from build123d import *
from build123d.topology import SkipClean

# Parameters (mm, degrees)
SKETCH1_W               = 112
SKETCH1_H               = 35.5
BOSS_EXTRUDE1_DEPTH     = 1
SKETCH2_W               = 6
SKETCH2_H               = 6
BOSS_EXTRUDE2_DEPTH     = 2
SKETCH3_R               = 1.1
CUT_EXTRUDE1_DEPTH      = 59.822295943
SKETCH4_R               = 2
CUT_EXTRUDE2_DEPTH      = 2
SKETCH5_W               = 20
SKETCH5_H               = 14
CUT_EXTRUDE3_DEPTH      = 59.822295943
CHAMFER1_SIZE           = 0.4
CUT_EXTRUDE4_DEPTH      = 0.2
SKETCH7_W               = 2.2
SKETCH7_H               = 2.2
CUT_EXTRUDE5_DEPTH      = 0.2
MIRROR2_COPY_1_DEPTH    = 0.2
MIRROR2_COPY_2_SKETCH_W = 2.2
MIRROR2_COPY_2_SKETCH_H = 2.2
MIRROR2_COPY_2_DEPTH    = 0.2
CUT_EXTRUDE6_DEPTH      = 59.779779687
CUT_EXTRUDE6_DEPTH_BACK = 59.779779687
SKETCH8_W               = 0.4
SKETCH8_H               = 35.5


with BuildPart() as part:
    # Sketch1 → Boss-Extrude1 (new body)
    with BuildSketch(Plane.XY):
        Rectangle(SKETCH1_W, SKETCH1_H)
    extrude(amount=BOSS_EXTRUDE1_DEPTH)

    # Sketch2 → Boss-Extrude2 (add)
    with BuildSketch(Plane.XY.offset(1)):
        with Locations((-53, 14.75)):
            Rectangle(SKETCH2_W, SKETCH2_H)
        with Locations((-53, -14.75)):
            Rectangle(SKETCH2_W, SKETCH2_H)
        with Locations((53, -14.75)):
            Rectangle(SKETCH2_W, SKETCH2_H)
        with Locations((53, 14.75)):
            Rectangle(SKETCH2_W, SKETCH2_H)
    extrude(amount=BOSS_EXTRUDE2_DEPTH)

    # Sketch3 → Cut-Extrude1 (cut, through all)
    with BuildSketch(Plane.XY.offset(3)):
        with Locations((-53, 14.75)):
            Circle(SKETCH3_R)
        with Locations(Location((-53, -14.75, 0), (0, 0, 180))):
            Circle(SKETCH3_R)
        with Locations((53, -14.75)):
            Circle(SKETCH3_R)
        with Locations(Location((53, 14.75, 0), (0, 0, 180))):
            Circle(SKETCH3_R)
    extrude(amount=-CUT_EXTRUDE1_DEPTH, mode=Mode.SUBTRACT)

    # Sketch4 → Cut-Extrude2 (cut)
    with BuildSketch(Plane(origin=(0, 0, 0), x_dir=(-1, 0, 0), z_dir=(0, 0, -1))):
        with Locations((-53, 14.75)):
            Circle(SKETCH4_R)
        with Locations((-53, -14.75)):
            Circle(SKETCH4_R)
        with Locations((53, 14.75)):
            Circle(SKETCH4_R)
        with Locations((53, -14.75)):
            Circle(SKETCH4_R)
    extrude(amount=-CUT_EXTRUDE2_DEPTH, mode=Mode.SUBTRACT)

    # Sketch5 → Cut-Extrude3 (cut, through all)
    with BuildSketch(Plane(origin=(0, 0, 0), x_dir=(-1, 0, 0), z_dir=(0, 0, -1))):
        with Locations((29.95, 6.75)):
            Rectangle(SKETCH5_W, SKETCH5_H)
    extrude(amount=-CUT_EXTRUDE3_DEPTH, mode=Mode.SUBTRACT)

    # Chamfer1
    chamfer1_edges = [part.edges().sort_by_distance(p)[0] for p in [
        (-39.95, 6.75, 0),
        (-29.95, 13.75, 0),
        (-19.95, 6.75, 0),
        (-29.95, -0.25, 0),
    ]]
    chamfer(chamfer1_edges, length=CHAMFER1_SIZE)

    # Sketch6 → Cut-Extrude4 (cut)
    with SkipClean():  # the faces are left unmerged after this step: merging them gives an invalid solid
        with BuildSketch(Plane(origin=(0, 0, 2), x_dir=(-1, 0, 0), z_dir=(0, 0, -1))):
            with BuildLine():
                Line((-54.1, 13.079670691), (-54.1, 16.420329309))
                ThreePointArc((-54.1, 16.420329309), (-53, 16.75), (-51.9, 16.420329309))
                Line((-51.9, 16.420329309), (-51.9, 13.079670691))
                ThreePointArc((-51.9, 13.079670691), (-53, 12.75), (-54.1, 13.079670691))
            make_face()
        cut_extrude4 = extrude(amount=-CUT_EXTRUDE4_DEPTH, mode=Mode.SUBTRACT)

    # Sketch7 → Cut-Extrude5 (cut)
    with SkipClean():  # the faces are left unmerged after this step: merging them gives an invalid solid
        with BuildSketch(Plane(origin=(0, 0, 2.2), x_dir=(-1, 0, 0), z_dir=(0, 0, -1))):
            with Locations((-53, 14.75)):
                Rectangle(SKETCH7_W, SKETCH7_H)
        cut_extrude5 = extrude(amount=-CUT_EXTRUDE5_DEPTH, mode=Mode.SUBTRACT)

    # Mirror1: Cut-Extrude4, Cut-Extrude5 across plane
    with SkipClean():  # the faces are left unmerged after this step: merging them gives an invalid solid
        add(cut_extrude4.mirror(Plane(origin=(0, 0, 0), x_dir=(0, 0, 1), z_dir=(1, 0, 0))), mode=Mode.SUBTRACT)
        add(cut_extrude5.mirror(Plane(origin=(0, 0, 0), x_dir=(0, 0, 1), z_dir=(1, 0, 0))), mode=Mode.SUBTRACT)

    # Mirror2: Cut-Extrude4, Cut-Extrude5 across plane
    with SkipClean():  # the faces are left unmerged after this step: merging them gives an invalid solid
        add(cut_extrude4.mirror(Plane.ZX), mode=Mode.SUBTRACT)
        add(cut_extrude5.mirror(Plane.ZX), mode=Mode.SUBTRACT)

    # Mirror2 copy 1 sketch → Mirror2 copy 1 (cut)
    with SkipClean():  # the faces are left unmerged after this step: merging them gives an invalid solid
        with BuildSketch(Plane(origin=(0, 0, 2), x_dir=(1, 0, 0), z_dir=(0, 0, -1))):
            with BuildLine():
                Line((-54.1, 13.079670691), (-54.1, 16.420329309))
                ThreePointArc((-54.1, 16.420329309), (-53, 16.75), (-51.9, 16.420329309))
                Line((-51.9, 16.420329309), (-51.9, 13.079670691))
                ThreePointArc((-51.9, 13.079670691), (-53, 12.75), (-54.1, 13.079670691))
            make_face()
        extrude(amount=-MIRROR2_COPY_1_DEPTH, mode=Mode.SUBTRACT)

    # Mirror2 copy 2 sketch → Mirror2 copy 2 (cut)
    with SkipClean():  # the faces are left unmerged after this step: merging them gives an invalid solid
        with BuildSketch(Plane(origin=(0, 0, 2.2), x_dir=(1, 0, 0), z_dir=(0, 0, -1))):
            with Locations((-53, 14.75)):
                Rectangle(MIRROR2_COPY_2_SKETCH_W, MIRROR2_COPY_2_SKETCH_H)
        extrude(amount=-MIRROR2_COPY_2_DEPTH, mode=Mode.SUBTRACT)

    # Sketch8 → Cut-Extrude6 (cut, two sides: drawn at the far end of the back side and taken through both)
    with SkipClean():  # the faces are left unmerged after this step: merging them gives an invalid solid
        with BuildSketch(Plane.XY.offset(1).offset(-CUT_EXTRUDE6_DEPTH_BACK)):
            with Locations((-55.8, 0)):
                Rectangle(SKETCH8_W, SKETCH8_H)
            with Locations((55.8, 0)):
                Rectangle(SKETCH8_W, SKETCH8_H)
        extrude(amount=CUT_EXTRUDE6_DEPTH + CUT_EXTRUDE6_DEPTH_BACK, mode=Mode.SUBTRACT)


solid = part.part
Could you check a few things on this model? Use its own coordinates, in mm. A direction names the side the tool comes from. Coordinates: 2 decimals unless noted, no trailing zeros. Order: outer loops, then holes, each group sorted by start corner. A loop starts at its lowest first (then second) coordinate and runs counter-clockwise, first axis right, second up. Notation, with made-up numbers: (50.25, -28) - (90.25, -28) arc R24 cw to (90.25, 2) - close; hole circle Ø6 at (8.5, 76.5). An arc over 180 degrees is marked (long way). Answer in a Markdown table with one row per item. Add a question column.
(1) If we section it at A-A, the plane x = -23: Please give me the cut outline in (y, z).
(2) If we mould it in two halves opening along Y, with no side actions, what happens to faces 4 (the face through (-13.1, -17.75, 0.8)), 5 (the face through (-51.6, -14.7, 3)), 6 (the face through (-53, 11.75, 2))? For each: released by +Y, released by -Y, zero draft, split by the parting line, or undercut.
(3) If we section it at C-C, the plane y = -4: Please give me the cut outline in (x, z).
(4) On a 3-axis mill with a long thin cutter (end or side, diameter ignored), from which of +Z, -Z, +X, -X, +Y, -Y can I reach the whole of each face in a straight line? I mean faces 1 (the face through (53, -11.75, 2)), 2 (the face through (55.6, -0.2, 0.8)), 3 (the face through (50, 15, 2)). Say none if no direction works.
(5) If we section it at D-D, the plane x = 25.5: Please give me the cut outline in (y, z).
(6) I need wall thicknesses on L1, parallel to Y at x = 53, z = 2.8; L2, parallel to Y at x = 53, z = 0.65; L3, parallel to Y at x = 53, z = 1.15. Which ranges of each line are inside material? Lowest first, please.
(7) Will these pins go through, and if not, where does the flat tip stop? pin 1 (0.5 mm diameter, centred on x = -52.5, y = -15.5, fed in from -Z); pin 2 (1.8 mm diameter, centred on x = 53, y = 14.75, fed in from +Z); pin 3 (2 mm diameter, centred on x = -42, y = -3.5, fed in from +Z); pin 4 (3 mm diameter, centred on x = 53, y = -14.75, fed in from -Z).
(8) If we section it at B-B, the plane y = 8: Please give me the cut outline in (x, z).
Results are:
| question | item | result |
|---|---|---|
| 1 | outline | (-17.75, 0) - (-0.65, 0) - (-0.25, 0.4) - (-0.25, 1) - (-17.75, 1) - close; (13.75, 0.4) - (14.15, 0) - (17.75, 0) - (17.75, 1) - (13.75, 1) - close |
| 2 | face 4 | released by -Y |
| 2 | face 5 | zero draft |
| 2 | face 6 | undercut |
| 3 | outline | (-55.6, 0) - (55.6, 0) - (55.6, 1) - (-55.6, 1) - close |
| 4 | face 1 | +Z, +X, -X |
| 4 | face 2 | +Z, -Z, +X, +Y, -Y |
| 4 | face 3 | +Z, +Y, -Y |
| 5 | outline | (-17.75, 0) - (17.75, 0) - (17.75, 1) - (-17.75, 1) - close |
| 6 | L1 | y = -17.75 to -15.85, -13.65 to -11.75, 11.75 to 13.65, 15.85 to 17.75 |
| 6 | L2 | y = -17.75 to -16.75, -12.75 to 12.75, 16.75 to 17.75 |
| 6 | L3 | y = -17.75 to -16.75, -12.75 to -11.75, 11.75 to 12.75, 16.75 to 17.75 |
| 7 | pin 1 | stops at z = 2.4 |
| 7 | pin 2 | passes through |
| 7 | pin 3 | stops at z = 1 |
| 7 | pin 4 | stops at z = 2 |
| 8 | outline | (-55.6, 0) - (-40.35, 0) - (-39.95, 0.4) - (-39.95, 1) - (-55.6, 1) - close; (-19.95, 0.4) - (-19.55, 0) - (55.6, 0) - (55.6, 1) - (-19.95, 1) - close |
